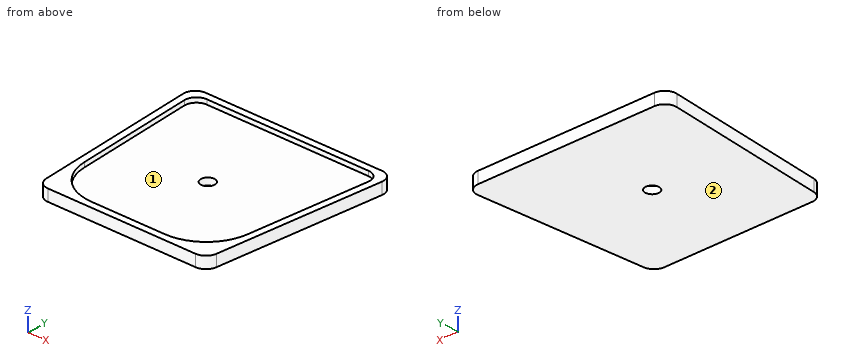
```python
from build123d import *

# Parameters (mm, degrees)
F1_DEPTH  = 10
F2_W      = 90
F2_H      = 40
F2_H_2    = 10
F3_DEPTH  = 10
F4_R      = 5
F5_R      = 4
F6_DEPTH  = 25
F7_R      = 3
F8_R      = 3
F10_DEPTH = 2
F11_R     = 3
F12_DEPTH = 25
F13_W     = 33.655686304
F13_H     = 120.6225939095
F14_DEPTH = 90.001
F15_R     = 5
F16_W     = 90.2396612329
F16_H     = 12.9153318724
F17_DEPTH = 50


with BuildPart() as f1:
    # F0 (on Top) → F1 (new body)
    with BuildSketch(Plane.XY):
        Polygon((41.5450818927, 0), (-48.4549181073, 0), (-40.9308930441, -86), (34.0210568295, -86), align=None)
    extrude(amount=F1_DEPTH)

    # F2 (on face) → F3 (join)
    with BuildSketch(Plane(origin=(0, 0, 0), x_dir=(-1, 0, 0), z_dir=(0, 1, 0))):
        with Locations((3.4549181073, 30)):
            Rectangle(F2_W, F2_H)
        with Locations((3.4549181073, 5)):
            Rectangle(F2_W, F2_H_2)
        with Locations((3.4549181073, -20)):
            Rectangle(F2_W, F2_H)
    extrude(amount=F3_DEPTH)

    # F4
    f4_edges = [f1.edges().sort_by_distance(p)[0] for p in [
        (-40.930893, -86, 5),
        (34.021057, -86, 5),
    ]]
    fillet(f4_edges, radius=F4_R)

    # F5 (on face) → F6 (cut)
    with BuildSketch(Plane.XZ):
        with Locations((-28.4549181073, 40)):
            Circle(F5_R)
        with Locations((21.5450818927, 40)):
            Circle(F5_R)
    extrude(amount=-F6_DEPTH, mode=Mode.SUBTRACT)

    # F7
    f7_edges = [f1.edges().sort_by_distance(p)[0] for p in [
        (-48.454918, 5, 50),
        (41.545082, 5, 50),
        (41.545082, 5, -40),
        (-48.454918, 5, -40),
    ]]
    fillet(f7_edges, radius=F7_R)

    # F8
    f8_edges = [f1.edges().sort_by_distance(p)[0] for p in [
        (-3.454918, 0, 10),
    ]]
    fillet(f8_edges, radius=F8_R)

    # F9 (on face) → F10 (cut)
    with BuildSketch(Plane.XY.offset(10)):
        with BuildLine():
            ThreePointArc((37.533121384, -11.4357787137), (36.2385345776, -7.6220489619), (32.5521478936, -6))
            Line((32.5521478936, -6), (-39.4619841082, -6))
            ThreePointArc((-39.4619841082, -6), (-43.1483707922, -7.6220489619), (-44.4429575986, -11.4357787137))
            Line((-44.4429575986, -11.4357787137), (-39.7791700035, -64.743114855))
            ThreePointArc((-39.7791700035, -64.743114855), (-33.367080194, -77.7455467362), (-19.8552760417, -83))
            Line((-19.8552760417, -83), (12.9454398271, -83))
            ThreePointArc((12.9454398271, -83), (26.4572439794, -77.7455467362), (32.8693337889, -64.743114855))
            Line((32.8693337889, -64.743114855), (37.533121384, -11.4357787137))
        make_face()
    extrude(amount=-F10_DEPTH, mode=Mode.SUBTRACT)

    # F11 (on face) → F12 (cut)
    with BuildSketch(Plane.XY.offset(8)):
        with Locations((-3.4549181073, -44.5)):
            Circle(F11_R)
    extrude(amount=-F12_DEPTH, mode=Mode.SUBTRACT)

    # F13 (on face) → F14 (cut, through all)
    with BuildSketch(Plane(origin=(-48.4549181073, 0, 0), x_dir=(0, -1, 0), z_dir=(-1, 0, 0))):
        with Locations((-13.827843152, 2.30451487)):
            Rectangle(F13_W, F13_H)
    extrude(amount=-F14_DEPTH, mode=Mode.SUBTRACT)

    # F15
    f15_edges = [f1.edges().sort_by_distance(p)[0] for p in [
        (-48.192452, -3, 5),
        (41.282616, -3, 5),
    ]]
    fillet(f15_edges, radius=F15_R)

    # F16 (on Right) → F17 (cut, symmetric)
    with BuildSketch(Plane.YZ):
        with Locations((-45.4951552674, -1.4576659362)):
            Rectangle(F16_W, F16_H)
    extrude(amount=F17_DEPTH, both=True, mode=Mode.SUBTRACT)


solid = f1.part
```
Input: part model. Units: mm. Frame: model coordinates. Face numbers are marked on the shaded views. A direction names the side the tool comes from. Round coordinates to 2 decimals unless told otherwise and drop trailing zeros. Loops run counter-clockwise (first coordinate to the right, second up) from the corner with the lowest first, then second, coordinate; pieces in that order, holes last. Notation, with made-up numbers: (-32, 73.5) -> (-28, 73.5) arc R20 ccw to (-28, 109.5) -> close; hole circle Ø9 at (41.5, 26). An arc over 180 degrees is marked (long way). One line per item, written item: value.
(1) Section A-A (z = 6.15). Return the cut outline in (x, y), plus the area to 3 significant figures.
Geometry check:
outline: (-47.72, -8.44) -> (-41.33, -81.44) arc R5 ccw to (-36.35, -86) -> (29.44, -86) arc R5 ccw to (34.42, -81.44) -> (40.81, -8.44) arc R5 ccw to (35.83, -3) -> (-42.74, -3) arc R5 ccw to start; hole circle Ø6 at (-3.45, -44.5)
area: 6,770 mm2
(2) Set-up query: the marked faces 1 and 2. Return all of +Z, -Z, +X, -X, +Y, -Y with unobstructed straight access to the full face (end or side cutting, diameter ignored); none if empty.
Geometry check:
face 1: +Z
face 2: -Z, +X, -X, +Y, -Y
(3) Section C-C (y = -57). Return the cut outline in (x, z).
Geometry check:
outline: (-43.47, 5) -> (36.56, 5) -> (36.56, 10) -> (33.55, 10) -> (33.55, 8) -> (-40.46, 8) -> (-40.46, 10) -> (-43.47, 10) -> close
(4) Material intervals for line 1 (Z direction, x = 33.5, y = -10); line 2 (Y direction, x = 9, z = 9.55); line 3 (X direction, y = -63.5, z = 8.3), sorted ascending. Write a range as [from, to].
Geometry check:
line 1: [5, 8]
line 2: [-86, -83], [-6, -3]
line 3: [-42.9, -39.89], [32.98, 35.99]
(5) Section D-D (y = -23). Return the cut outline in (x, z).
Geometry check:
outline: (-46.44, 5) -> (39.53, 5) -> (39.53, 10) -> (36.52, 10) -> (36.52, 8) -> (-43.43, 8) -> (-43.43, 10) -> (-46.44, 10) -> close
(6) Section B-B (y = -44.5). Return the cut outline in (x, z), plus the area to 3 significant figures.
Geometry check:
outline: (-44.56, 5) -> (-6.45, 5) -> (-6.45, 8) -> (-41.55, 8) -> (-41.55, 10) -> (-44.56, 10) -> close; (-0.45, 5) -> (37.65, 5) -> (37.65, 10) -> (34.64, 10) -> (34.64, 8) -> (-0.45, 8) -> close
area: 241 mm2
(7) Pin query (flat end, axial travel): pin 1 (1.5 mm diameter, centred on x = 12, y = -72.5, fed in from +Z); pin 2 (2 mm diameter, centred on y = -63, z = 8.5, fed in from -X); pin 3 (1 mm diameter, centred on y = -20, z = 6, fed in from +X). Return the tip coordinate at first contact, or that it passes through.
Geometry check:
pin 1: z = 8
pin 2: x = -43.03
pin 3: x = 39.84
